from build123d import *

# Parameters (mm, degrees)
BOSS_EXTRUDE1_DEPTH             = 4
FILLET1_R                       = 2
F_3_0MM_DOWEL_HOLE1_D           = 3
F_3_0MM_DOWEL_HOLE1_CSINK_D     = 3.05
F_3_0MM_DOWEL_HOLE1_CSINK_ANGLE = 90
SKETCH4_W                       = 4
SKETCH4_H                       = 18.1
BOSS_EXTRUDE2_DEPTH             = 42
CHAMFER1_SIZE                   = 4
FILLET2_R                       = 2
F_4_0MM_DOWEL_HOLE1_D           = 4
F_4_0MM_DOWEL_HOLE1_CSINK_D     = 4.05
F_4_0MM_DOWEL_HOLE1_CSINK_ANGLE = 90
CUT_EXTRUDE1_DEPTH              = 28
CUT_EXTRUDE1_DEPTH_BACK         = 5
CUT_EXTRUDE2_DEPTH              = 28
CUT_EXTRUDE2_DEPTH_BACK         = 5


with BuildPart() as part:
    # Sketch1 → Boss-Extrude1 (new body)
    with BuildSketch(Plane(origin=(0, 0, 0), x_dir=(1, 0, 0), z_dir=(0, 1, 0))):
        Polygon((0, 16.05), (0, -16.05), (8, -16.05), (8, -9.05), (31, -9.05), (31, 9.05), (8, 9.05), (8, 16.05), align=None)
    extrude(amount=BOSS_EXTRUDE1_DEPTH)

    # Fillet1
    fillet1_edges = [part.edges().sort_by_distance(p)[0] for p in [
        (8, 2, -16.05),
        (8, 2, -9.05),
        (8, 2, 9.05),
        (8, 2, 16.05),
        (0, 2, 16.05),
        (0, 2, -16.05),
    ]]
    fillet(fillet1_edges, radius=FILLET1_R)

    # Ø3.0mm Dowel Hole1 (through all)
    with Locations(Plane(origin=(0, 4, 0), x_dir=(1, 0, 0), z_dir=(0, 1, 0))):
        with Locations((4, 12.05), (4, -12.05)):
            CounterSinkHole(F_3_0MM_DOWEL_HOLE1_D / 2, F_3_0MM_DOWEL_HOLE1_CSINK_D / 2, counter_sink_angle=F_3_0MM_DOWEL_HOLE1_CSINK_ANGLE)

    # Sketch4 → Boss-Extrude2 (add)
    with BuildSketch(Plane(origin=(0, 0, 0), x_dir=(-1, 0, 0), z_dir=(0, -1, 0))):
        with Locations((-29, 0)):
            Rectangle(SKETCH4_W, SKETCH4_H)
    extrude(amount=BOSS_EXTRUDE2_DEPTH)

    # Chamfer1
    chamfer1_edges = [part.edges().sort_by_distance(p)[0] for p in [
        (27, 0, 0),
    ]]
    chamfer(chamfer1_edges, length=CHAMFER1_SIZE)

    # Fillet2
    fillet2_edges = [part.edges().sort_by_distance(p)[0] for p in [
        (31, 4, 0),
    ]]
    fillet(fillet2_edges, radius=FILLET2_R)

    # Ø4.0mm Dowel Hole1 (through all)
    with Locations(Plane(origin=(31, 0, 0), x_dir=(0, 0, -1), z_dir=(1, 0, 0))):
        with Locations((0, -36), (0, -27), (0, -18)):
            CounterSinkHole(F_4_0MM_DOWEL_HOLE1_D / 2, F_4_0MM_DOWEL_HOLE1_CSINK_D / 2, counter_sink_angle=F_4_0MM_DOWEL_HOLE1_CSINK_ANGLE)

    # Sketch11 → Cut-Extrude1 (cut, two sides)
    with BuildSketch(Plane.ZY.offset(-27)) as cut_extrude1_sk:
        Polygon((-9.05, -4), (-5.5, -13), (-5.5, -42), (-9.05, -42), align=None)
    extrude(amount=CUT_EXTRUDE1_DEPTH, mode=Mode.SUBTRACT)
    extrude(cut_extrude1_sk.sketch, amount=-CUT_EXTRUDE1_DEPTH_BACK, mode=Mode.SUBTRACT)

    # Sketch12 → Cut-Extrude2 (cut, two sides)
    with BuildSketch(Plane.ZY.offset(-27)) as cut_extrude2_sk:
        Polygon((9.05, -4), (5.5, -13), (5.5, -42), (9.05, -42), align=None)
    extrude(amount=CUT_EXTRUDE2_DEPTH, mode=Mode.SUBTRACT)
    extrude(cut_extrude2_sk.sketch, amount=-CUT_EXTRUDE2_DEPTH_BACK, mode=Mode.SUBTRACT)


solid = part.part
CAD build for the part. Positions are in the model's coordinates, mm. A direction names the side the tool comes from. Round coordinates to 2 decimals unless told otherwise and drop trailing zeros. Write each loop counter-clockwise with the first axis right and the second up, starting at its lowest first coordinate (ties: lowest second). Pieces come first, ordered by that corner, then holes. Notation, with made-up numbers: M 37.25,41.5 L 56.25,41.5 A9 ccw 56.25,58.5 Z; hole C -39.5,79 d6. An arc over 180 degrees is marked long. Use a Markdown table: item, result. Add a question column.
1. Slice it at D-D on z = -4.5. Give the cut face in (x, y), then the cut area to 3 significant figures.
2. Pull direction Z, two halves, no side cores. Call faces 3 (the face through (0.57, 2.03, 15.45)), 4 (the face through (29, -27, -5.5)), 5 (the face through (27, -19, 2)), 6 (the face through (4.325, 1.96, -10.586)): released by +Z, released by -Z, zero draft, split by the parting line, or undercut.
3. Drill centre lines: probe 1 along Z at (x, y) = (28, -36); probe 2 along Y at (x, z) = (27.9, 0); probe 3 along Y at (x, z) = (3.5, -3.5). Where is each one in solid material? Low to high.
4. Flat gauge pins, fed straight in: P1, Ø12, axis at y = -11, z = 6.5, coming from the -X side; P2, Ø2, axis at x = 30, y = -30.5, coming from the -Z side; P3, Ø2.5, axis at x = 25, y = -1.5, coming from the -Z side. Where does each tip first touch, or does it go through?
5. Slice it at B-B on y = -18. Give the cut face in (x, z) (3 decimals), then the cut area to 3 significant figures.
6. Slice it at C-C on z = 12.05. Give the cut face in (x, y) (3 decimals), then the cut area to 3 significant figures.
7. 3-axis set-ups, long thin cutter, end or side, ignore diameter. For faces 1 (the face through (8, 2, 13)), 2 (the face through (25, -2, 0)): which of +Z, -Z, +X, -X, +Y, -Y reach the whole face in a straight line?
8. Slice it at A-A on z = 0. Give the cut face in (x, y) (3 decimals).
Reply:
| question | item | result |
|---|---|---|
| 1 | outline | M 0,0 L 23,0 L 27,-4 L 27,-42 L 31,-42 L 31,2 A2 ccw 29,4 L 0,4 Z |
| 1 | area | 299 mm^2 |
| 2 | face 3 | released by +Z |
| 2 | face 4 | released by -Z |
| 2 | face 5 | zero draft |
| 2 | face 6 | undercut |
| 3 | probe 1 | z = -5.5 to -2, 2 to 5.5 |
| 3 | probe 2 | y = -42 to -38, -34 to -29, -25 to -20, -16 to 4 |
| 3 | probe 3 | y = 0 to 4 |
| 4 | P1 | stops at x = 27 |
| 4 | P2 | stops at z = -5.5 |
| 4 | P3 | stops at z = -9.05 |
| 5 | outline | M 27,-5.5 L 31,-5.5 L 31,-2.025 L 30.975,-2 L 27,-2 Z; M 27,2 L 30.975,2 L 31,2.025 L 31,5.5 L 27,5.5 Z |
| 5 | area | 28.0 mm^2 |
| 6 | outline | M 0,0 L 2.5,0 L 2.5,3.975 L 2.475,4 L 0,4 Z; M 5.5,0 L 8,0 L 8,4 L 5.525,4 L 5.5,3.975 Z |
| 6 | area | 20.0 mm^2 |
| 7 | face 1 | +Z, +X, +Y, -Y |
| 7 | face 2 | +Z, -Z, -X, -Y |
| 8 | outline | M 0,0 L 23,0 L 27,-4 L 27,-16 L 30.975,-16 L 31,-15.975 L 31,2 A2 ccw 29,4 L 0,4 Z; M 27,-42 L 31,-42 L 31,-38.025 L 30.975,-38 L 27,-38 Z; M 27,-34 L 30.975,-34 L 31,-33.975 L 31,-29.025 L 30.975,-29 L 27,-29 Z; M 27,-25 L 30.975,-25 L 31,-24.975 L 31,-20.025 L 30.975,-20 L 27,-20 Z |
